from build123d import *

# Parameters (mm, degrees)
CROQUIS1_R              = 1.25
SALIENTE_EXTRUIR1_DEPTH = 1.5
SALIENTE_EXTRUIR2_DEPTH = 55
CORTAR_EXTRUIR1_DEPTH   = 17.5
CORTAR_EXTRUIR2_DEPTH   = 17.5
CROQUIS4_R              = 1.5
CORTAR_EXTRUIR3_DEPTH   = 2.049041
SALIENTE_EXTRUIR3_DEPTH = 4


with BuildPart() as part:
    # Croquis1 → Saliente-Extruir1 (new body)
    with BuildSketch(Plane.XY):
        Polygon((-68.837310195, 14.25), (-55.837310195, 14.25), (-45.737310195, 24.35), (-36.937310195, 24.35), (-26.837310195, 14.25), (-13.837310195, 14.25), (-13.837310195, 4.25), (-68.837310195, 4.25), align=None)
        with Locations((-18.087310195, 10.5)):
            Circle(CROQUIS1_R, mode=Mode.SUBTRACT)
        with Locations((-64.587310195, 10.5)):
            Circle(CROQUIS1_R, mode=Mode.SUBTRACT)
    extrude(amount=SALIENTE_EXTRUIR1_DEPTH)

    # Croquis2 → Saliente-Extruir2 (add)
    with BuildSketch(Plane.ZY.offset(68.837310195)):
        Polygon((13.856406461, -3.75), (14.880925513, -1.975480947), (1.5, 5.75), (1.5, 4.25), (0, 4.25), align=None)
    extrude(amount=-SALIENTE_EXTRUIR2_DEPTH)

    # Croquis2<2> → Cortar-Extruir1 (cut)
    with BuildSketch(Plane.ZY.offset(68.837310195)):
        Polygon((13.856406461, -3.75), (14.880925513, -1.975480947), (1.5, 5.75), (1.5, 4.25), (0, 4.25), align=None)
    extrude(amount=-CORTAR_EXTRUIR1_DEPTH, mode=Mode.SUBTRACT)

    # Croquis3 → Cortar-Extruir2 (cut)
    with BuildSketch(Plane(origin=(-13.837310195, 0, 0), x_dir=(0, 0, -1), z_dir=(1, 0, 0))):
        Polygon((-1.5, 5.75), (-14.880925513, -1.975480947), (-13.856406461, -3.75), (0, 4.25), (-1.5, 4.25), align=None)
    extrude(amount=-CORTAR_EXTRUIR2_DEPTH, mode=Mode.SUBTRACT)

    # Croquis4 → Cortar-Extruir3 (cut)
    with BuildSketch(Plane(origin=(0, 3.1875, 1.840303983), x_dir=(1, 0, 0), z_dir=(0, -0.8660254037844399, -0.4999999999999978))):
        with Locations(Location((-36.337310195, 9.875, 0), (0, 0, 270))):
            Circle(CROQUIS4_R)
        with Locations(Location((-46.337310195, 9.875, 0), (0, 0, 270))):
            Circle(CROQUIS4_R)
    extrude(amount=-CORTAR_EXTRUIR3_DEPTH, mode=Mode.SUBTRACT)

    # Croquis5 → Saliente-Extruir3 (add)
    with BuildSketch(Plane.XZ.offset(-4.25)):
        Polygon((-26.454313708, 1.5), (-24.454313708, 1.5), (-24.454313708, 3.3), (-21.454313708, 3.3), (-21.454313708, 1.5), (-19.454313708, 1.5), (-19.454313708, 5.3), (-26.454313708, 5.3), align=None)
    extrude(amount=-SALIENTE_EXTRUIR3_DEPTH)


solid = part.part
The model under review builds one solid part; all positions refer to its coordinate system, in mm. A direction names the side the tool comes from. Round coordinates to 2 decimals unless told otherwise and drop trailing zeros. Order: outer loops, then holes, each group sorted by start corner. A loop starts at its lowest first (then second) coordinate and runs counter-clockwise, first axis right, second up. Notation, with made-up numbers: (49.5, 26.5) - (89.5, 26.5) arc R12 cw to (89.5, 42.5) - close; hole circle Ø11 at (63.5, 0). An arc over 180 degrees is marked (long way). Use one line per item in the form item = value.
Q1. Clearance check with flat-ended pins moving along their axes: P1, Ø1.6, axis at x = -61, z = 1, coming from the +Y side; P2, Ø5, axis at x = -44, z = 7.5, coming from the -Y side; P3, Ø1.4, axis at y = 7, z = 2.5, coming from the -X side; P4, Ø0.9, axis at x = -23, y = 5.5, coming from the -Z side. State where each tip first meets the part, or that it passes through.
Response values:
P1 = 14.25
P2 = -1.52
P3 = -26.45
P4 = 0
Q2. Add section D-D on z = 7. Give the boundary of the cut face in (x, y).
Response values:
outline = (-51.34, 0.21) - (-31.34, 0.21) - (-31.34, 2.57) - (-51.34, 2.57) - close
Q3. To check wall thickness, follow line 1 (Z direction, x = -25.5, y = 13.75); line 2 (Y direction, x = -58.5, z = 1.25); line 3 (Z direction, x = -19.5, y = 7). State the ranges of each line that lie inside material, in increasing order.
Response values:
line_1 = 0 to 1.5
line_2 = 4.25 to 14.25
line_3 = 0 to 5.3
Q4. Add section B-B on x = -43. Give the boundary of the cut face in (y, z).
Response values:
outline = (-3.75, 13.86) - (4.25, 0) - (24.35, 0) - (24.35, 1.5) - (5.75, 1.5) - (-1.98, 14.88) - close
Q5. Mouldability with a two-part tool opening along Z and no side actions: class faces 5 (the flat face through (-41.477, 1.833, 8.284)), 6 (the cylindrical face through (-44.85, -0.97, 11.07)), 7 (the flat face through (-62, 14.25, 1)) as pulls with the +Z half, pulls with the -Z half, needs draft (parallel to the pull), parting line crosses it, or undercut.
Response values:
face_5 = pulls with the +Z half
face_6 = undercut
face_7 = needs draft
Q6. Add section C-C on y = 18.75. Give the boundary of the cut face in (x, z).
Response values:
outline = (-51.34, 0) - (-31.34, 0) - (-31.34, 1.5) - (-51.34, 1.5) - close
Q7. Tool access review of faces 1 (the flat face through (-20, 14.25, 1)), 2 (the flat face through (-23, 8.25, 4)), 3 (the flat face through (-24.454, 6, 2)), 4 (the flat face through (-22, 4.25, 1)): name each direction out of +Z, -Z, +X, -X, +Y, -Y from which nothing blocks a thin tool from reaching the whole face with its end or side.
Response values:
face_1 = +Z, -Z, +X, +Y
face_2 = +Z, +X, -X, +Y
face_3 = +Y, -Y
face_4 = +Z, -Z, +X, -Y
Q8. Add section A-A on y = 10.5. Give the boundary of the cut face in (x, z), then the cut area to 3 significant figures.
Response values:
outline = (-68.84, 0) - (-65.84, 0) - (-65.84, 1.5) - (-68.84, 1.5) - close; (-63.34, 0) - (-19.34, 0) - (-19.34, 1.5) - (-63.34, 1.5) - close; (-16.84, 0) - (-13.84, 0) - (-13.84, 1.5) - (-16.84, 1.5) - close
area = 75.0 mm^2
